Could you check a few things on this model? Use its own coordinates, in mm. A direction names the side the tool comes from. Coordinates: 2 decimals unless noted, no trailing zeros. Write each loop counter-clockwise with the first axis right and the second up, starting at its lowest first coordinate (ties: lowest second). Pieces come first, ordered by that corner, then holes.
```python
from build123d import *

# Parameters (mm, degrees)
SKETCH1_R           = 20
BOSS_EXTRUDE1_DEPTH = 4
SKETCH2_R           = 16.5
CUT_EXTRUDE1_DEPTH  = 1.5
CHAMFER1_SIZE       = 1.5


with BuildPart() as part:
    # Sketch1 → Boss-Extrude1 (new body)
    with BuildSketch(Plane(origin=(0, 0, 0), x_dir=(1, 0, 0), z_dir=(0, 1, 0))):
        Circle(SKETCH1_R)
    extrude(amount=BOSS_EXTRUDE1_DEPTH)

    # Sketch2 → Cut-Extrude1 (cut)
    with BuildSketch(Plane(origin=(0, 4, 0), x_dir=(1, 0, 0), z_dir=(0, 1, 0))):
        Circle(SKETCH2_R)
    extrude(amount=-CUT_EXTRUDE1_DEPTH, mode=Mode.SUBTRACT)

    # Chamfer1
    chamfer1_edges = [part.edges().sort_by_distance(p)[0] for p in [
        (-20, 0, 0),
    ]]
    chamfer(chamfer1_edges, length=CHAMFER1_SIZE)


solid = part.part
```
Item 1: If I drill on line 1 along Z through (x, y) = (0, 3.45); line 2 along Y through (x, z) = (0, 6.5), over which ranges is the centre line in solid material (lowest first)?
Item 2: I want a section at A-A, the plane z = 0. List the corners of the cut face in (x, y) for me, then the cut area to 3 significant figures.
Item 3: I want a section at C-C, the plane y = 3.4. List the corners of the cut face in (x, z) for me, then the cut area to 3 significant figures.
Item 4: If we mould it in two halves opening along Z, with no side actions, what happens to faces 1 (the flat face through (0, 0, 0)), 2 (the cylindrical face through (-4.336, 2.732, 19.524)), 3 (the flat face through (0, 2.5, 0))? For each: released by +Z, released by -Z, zero draft, split by the parting line, or undercut.
Item 5: Which directions (+Z, -Z, +X, -X, +Y, -Y) give clear straight access to the entire face, cutting with the end or side of a thin tool? Please do faces 4 (the flat face through (2.9, 4, -16.4)), 5 (the cylindrical face through (15.24, 3.26, 6.32)).
Item 6: I want a section at B-B, the plane x = 0. List the corners of the cut face in (y, z) for me, then the cut area to 3 significant figures.
Item 7: Will these pins go through, and if not, where does the flat tip stop? pin 1 Ø10 at (x, z) = (3.5, 0) entering from +Y; pin 2 Ø1 at (y, z) = (3, 6.5) entering from -X; pin 3 Ø2 at (y, z) = (3.5, 4.5) entering from +X.
Taken from the geometry:
1. line 1: z = -20 to -16.5, 16.5 to 20
1. line 2: y = 0 to 2.5
2. outline: (-20, 1.5) - (-18.5, 0) - (18.5, 0) - (20, 1.5) - (20, 4) - (16.5, 4) - (16.5, 2.5) - (-16.5, 2.5) - (-16.5, 4) - (-20, 4) - close
2. area: 108 mm2
3. outline: circle Ø40 at (0, 0); hole circle Ø33 at (0, 0)
3. area: 401 mm2
4. face 1: zero draft
4. face 2: split by the parting line
4. face 3: undercut
5. face 4: +Z, -Z, +X, -X, +Y
5. face 5: +Y
6. outline: (0, -18.5) - (1.5, -20) - (4, -20) - (4, -16.5) - (2.5, -16.5) - (2.5, 16.5) - (4, 16.5) - (4, 20) - (1.5, 20) - (0, 18.5) - close
6. area: 108 mm2
7. pin 1: stops at y = 2.5
7. pin 2: stops at x = -19.08
7. pin 3: stops at x = 19.69
